from build123d import *

# Parameters (mm, degrees)
F3_DEPTH = 4
F0_R     = 1.75
F4_DEPTH = 2


with BuildPart() as f2:
    # F2: sweep along a path in F1
    with BuildLine(Plane.XZ) as f2_path:
        Line((0, 0), (6.840403, 18.793852))
    # F0 (on Top) → F2 (sweep)
    with BuildSketch(Plane.XY):
        Polygon((-17.171573, 33.579285), (-20, 33.579285), (-20, -26.420715), (-17.171573, -26.420715), (-18, -25.592288), (-18, 32.750857), align=None)
    sweep(path=f2_path.line)

    # F0 (on Top) → F3 (join)
    with BuildSketch(Plane.XY):
        Polygon((-8, 33.579285), (-17.171573, 33.579285), (-18, 32.750857), (-18, -25.592288), (-17.171573, -26.420715), (-8, -26.420715), align=None)
        Polygon((-13, -13.245289), (-10.25, -14.833002), (-10.25, -18.008429), (-13, -19.596142), (-15.75, -18.008429), (-15.75, -14.833002), align=None, mode=Mode.SUBTRACT)
        Polygon((-13, 6.754711), (-10.25, 5.166998), (-10.25, 1.991571), (-13, 0.403858), (-15.75, 1.991571), (-15.75, 5.166998), align=None, mode=Mode.SUBTRACT)
        Polygon((-13, 26.754711), (-10.25, 25.166998), (-10.25, 21.991571), (-13, 20.403858), (-15.75, 21.991571), (-15.75, 25.166998), align=None, mode=Mode.SUBTRACT)
    extrude(amount=F3_DEPTH)

    # F0 (on Top) → F4 (join)
    with BuildSketch(Plane.XY):
        Polygon((-10.25, 21.991571), (-10.25, 25.166998), (-13, 26.754711), (-15.75, 25.166998), (-15.75, 21.991571), (-13, 20.403858), align=None)
        with Locations((-13, 23.579285)):
            Circle(F0_R, mode=Mode.SUBTRACT)
        Polygon((-10.25, 1.991571), (-10.25, 5.166998), (-13, 6.754711), (-15.75, 5.166998), (-15.75, 1.991571), (-13, 0.403858), align=None)
        with Locations((-13, 3.579285)):
            Circle(F0_R, mode=Mode.SUBTRACT)
        Polygon((-10.25, -18.008429), (-10.25, -14.833002), (-13, -13.245289), (-15.75, -14.833002), (-15.75, -18.008429), (-13, -19.596142), align=None)
        with Locations((-13, -16.420715)):
            Circle(F0_R, mode=Mode.SUBTRACT)
    extrude(amount=F4_DEPTH)


solid = f2.part
Work out the finished part from the listing and answer in its coordinate system (mm). A direction names the side the tool comes from. Give positions to 0.01 mm unless a question says otherwise; leave off trailing zeros. Loops run counter-clockwise (first coordinate to the right, second up) from the corner with the lowest first, then second, coordinate; pieces in that order, holes last. Notation, with made-up numbers: (16, -38.5) -> (22, -38.5) arc R12 cw to (22, -18.5) -> close; hole circle Ø6 at (34.5, -23). An arc over 180 degrees is marked (long way). Use a Markdown table: item, result. Add a question column.
1) Consider line 1 along Y through (x, z) = (-13, 0.4); line 2 along Z through (x, y) = (-8.75, 14.5); line 3 along X through (y, z) = (-13, 8.5). Determine where each line is inside the solid, lowest interval first.
2) For a pull along X with two mould halves and no side action, classify faces 4 (the flat face through (-11.606, -18.791, 2.986)), 5 (the flat face through (-13.6, 33, 11.4)) as +X half, -X half, draft (parallel to the pull), parting line (faces both ways), or undercut.
3) Which of the six approach directions +Z, -Z, +X, -X, +Y, -Y give full straight-line access (tool end or side, diameter ignored) to faces 1 (the flat face through (-10.25, -16, 3)), 2 (the cylindrical face through (-11.383, -17.091, 0.986)), 3 (the flat face through (-15.75, 4, 3))?
4) Each of these flat-tipped pins is pushed along its axis until it touches: P1, Ø1, axis at y = 3.5, z = 2.5, coming from the -X side; P2, Ø5, axis at y = 2.5, z = 9.5, coming from the -X side; P3, Ø3, axis at y = -5.5, z = 4.5, coming from the -X side. Where does it stop, or does it pass through?
5) The part is cut by section D-D, the plane z = 3.25. Determine the outline of the cut face in (x, y), plus the area to 3 significant figures.
6) The part is cut by section B-B, the plane y = 23. Determine the outline of the cut face in (x, z).
7) The part is cut by section A-A, the plane x = -13.75. Count the separate pieces of the cut face and the enclosed holes in it, plus the area to 3 significant figures.
8) The part is cut by section C-C, the plane y = -8.5. Determine the outline of the cut face in (x, z), plus the area to 3 significant figures.
Reported:
| question | item | result |
|---|---|---|
| 1 | line 1 | y = -26.42 to -18.17, -14.67 to 1.83, 5.33 to 21.83, 25.33 to 33.58 |
| 1 | line 2 | z = 0 to 4 |
| 1 | line 3 | x = -16.91 to -14.91 |
| 2 | face 4 | undercut |
| 2 | face 5 | +X half |
| 3 | face 1 | +Z |
| 3 | face 2 | -Z |
| 3 | face 3 | none |
| 4 | P1 | stops at x = -19.27 |
| 4 | P2 | stops at x = -17.45 |
| 4 | P3 | stops at x = -18.91 |
| 5 | outline | (-18.82, -26.42) -> (-8, -26.42) -> (-8, 33.58) -> (-18.82, 33.58) -> close; hole (-15.75, -18.01) -> (-13, -19.6) -> (-10.25, -18.01) -> (-10.25, -14.83) -> (-13, -13.25) -> (-15.75, -14.83) -> close; hole (-15.75, 1.99) -> (-13, 0.4) -> (-10.25, 1.99) -> (-10.25, 5.17) -> (-13, 6.75) -> (-15.75, 5.17) -> close; hole (-15.75, 21.99) -> (-13, 20.4) -> (-10.25, 21.99) -> (-10.25, 25.17) -> (-13, 26.75) -> (-15.75, 25.17) -> close |
| 5 | area | 570 mm^2 |
| 6 | outline | (-20, 0) -> (-14.65, 0) -> (-14.65, 2) -> (-15.75, 2) -> (-15.75, 4) -> (-16.54, 4) -> (-11.16, 18.79) -> (-13.16, 18.79) -> close; (-11.35, 0) -> (-8, 0) -> (-8, 4) -> (-10.25, 4) -> (-10.25, 2) -> (-11.35, 2) -> close |
| 7 | separate pieces | 5 |
| 7 | enclosed holes | 0 |
| 7 | area | 520 mm^2 |
| 8 | outline | (-20, 0) -> (-8, 0) -> (-8, 4) -> (-16.54, 4) -> (-11.16, 18.79) -> (-13.16, 18.79) -> close |
| 8 | area | 74.7 mm^2 |
